Autodesk Inventor part; units mm, degrees
ref_plane "YZ Plane" through (0, 0, 0) normal (1, 0, 0) x (0, 1, 0)
ref_plane "XZ Plane" through (0, 0, 0) normal (0, 1, 0) x (-1, 0, 0)
ref_plane "XY Plane" through (0, 0, 0) normal (0, 0, 1) x (1, 0, 0)
sketch "Sketch1" plane through (0, 0, 0) normal (1, 0, 0) x (0, 1, 0)
  line L0 (-5, 40.398) -> (-5, 37.398)
  line L1 (-5, 37.398) -> (5, 37.398)
  line L2 (5, 37.398) -> (5, 40.398)
  line L3 (-21, 40.398) -> (-5, 40.398)
  line L4 (5, 40.398) -> (21, 40.398)
  line L5 (-21, 40.398) -> (-21, 40.6202)
  line L6 (21, 40.398) -> (21, 40.6202)
  arc A0 (-20.7253, 41.0666) -> (-21, 40.6202) centre (-20.5, 40.6202) ccw
  arc A1 (21, 40.6202) -> (20.7253, 41.0666) centre (20.5, 40.6202) ccw
  arc A2 (20.7253, 41.0666) -> (-20.7253, 41.0666) centre (0, 0) ccw
  point P0 (0, 37.398)
  dimension "d3" = 10
  dimension "d6" = 3
  dimension "d7" = 42
  dimension "d8" = 16
  dimension "d9" = 0.5
  dimension "d10" = 37.398
extrude "Extrusion1" add sketch "Sketch1" along normal blind 3
properties part number "Camera Blinder 25090213"
Verification items for the finished model (mm, model axes). A direction names the side the tool comes from. Coordinates: 2 decimals unless noted, no trailing zeros. Write each loop counter-clockwise with the first axis right and the second up, starting at its lowest first coordinate (ties: lowest second). Pieces come first, ordered by that corner, then holes. Notation, with made-up numbers: M -29,-9 L -9,-9 A11 ccw -9,-5 Z; hole C 78,72.5 d11. An arc over 180 degrees is marked long. One line per item, written item: value.
Item 1: Scan lines: line 1 along Y through (x, z) = (2.8, 38.5); line 2 along Z through (x, y) = (0.4, -14.5); line 3 along Z through (x, y) = (1.45, -12.5). Record each from-to range of solid material in increasing order.
Check sheet entries:
line 1: y = -5 to 5
line 2: z = 40.4 to 43.65
line 3: z = 40.4 to 44.27
Item 2: Access from +Z, -Z, +X, -X, +Y, -Y to the whole of each face (thin tool, end or side, straight path). Record for faces 1 (the flat face through (1, 5, 39)), 2 (the flat face through (1, -5, 39)), 3 (the cylindrical face through (1, 0, 46)).
Check sheet entries:
face 1: -Z, +X, -X, +Y
face 2: -Z, +X, -X, -Y
face 3: +Z, +X, -X
Item 3: Section check B-B, the plane y = 4. Record the boundary of the cut face in (x, z).
Check sheet entries:
outline: M 0,37.4 L 3,37.4 L 3,45.83 L 0,45.83 Z
Item 4: Gauge pin test, flat end, axial feed: pin 1 Ø0.9 at (x, y) = (2, 10.5) entering from -Z. Record the tip position at first contact, or that the pin passes through.
Check sheet entries:
pin 1: stops at z = 40.4
Item 5: Section check C-C, the plane z = 45. Record the boundary of the cut face in (x, y).
Check sheet entries:
outline: M 0,-9.54 L 3,-9.54 L 3,9.54 L 0,9.54 Z
Item 6: Section check A-A, the plane x = 0.8. Record the boundary of the cut face in (y, z).
Check sheet entries:
outline: M -21,40.4 L -5,40.4 L -5,37.4 L 5,37.4 L 5,40.4 L 21,40.4 L 21,40.62 A0.5 ccw 20.73,41.07 A46 ccw -20.73,41.07 A0.5 ccw -21,40.62 Z
